Verification items for this drawing (mm, ordinates from the low corner). A direction names the side the tool comes from. Round coordinates to 2 decimals unless told otherwise and drop trailing zeros. Order: outer loops, then holes, each group sorted by start corner. A loop starts at its lowest first (then second) coordinate and runs counter-clockwise, first axis right, second up. Notation, with made-up numbers: (65, -15.5) - (89, -15.5) arc R23 ccw to (89, 15.5) - close; hole circle Ø3 at (-1, 60.25). An arc over 180 degrees is marked (long way). Return JSON: item names as keys, results as strings. Group by question number.
Q1. Material ranges on line 1 along Y through (x, z) = (3.75, 0.8); line 2 along X through (y, z) = (3.5, 1.4); line 3 along X through (y, z) = (12, 1.25), recorded low to high.
Q2. Sectioned sample at C-C, the plane y = 2.5. Record the cut outline in (x, z), then the cut area to 3 significant figures.
Q3. Sectioned sample at B-B, the plane x = 3. Record the cut outline in (y, z).
Q4. Sectioned sample at A-A, the plane z = 1.6. Record the cut outline in (x, y), then the cut area to 3 significant figures.
Q5. Tool access check on the marked faces 1, 2 and 3. Record the directions out of +Z, -Z, +X, -X, +Y, -Y that give a thin tool (end or side, any length) a straight path to the whole face; none if there is none.
Q6. Gauge pin test, flat ends, axial feed: pin 1 Ø0.6 at (y, z) = (2, 1) entering from +X; pin 2 Ø1.5 at (x, y) = (9.5, 4) entering from -Z. Record the tip position at first contact, or that the pin passes through.
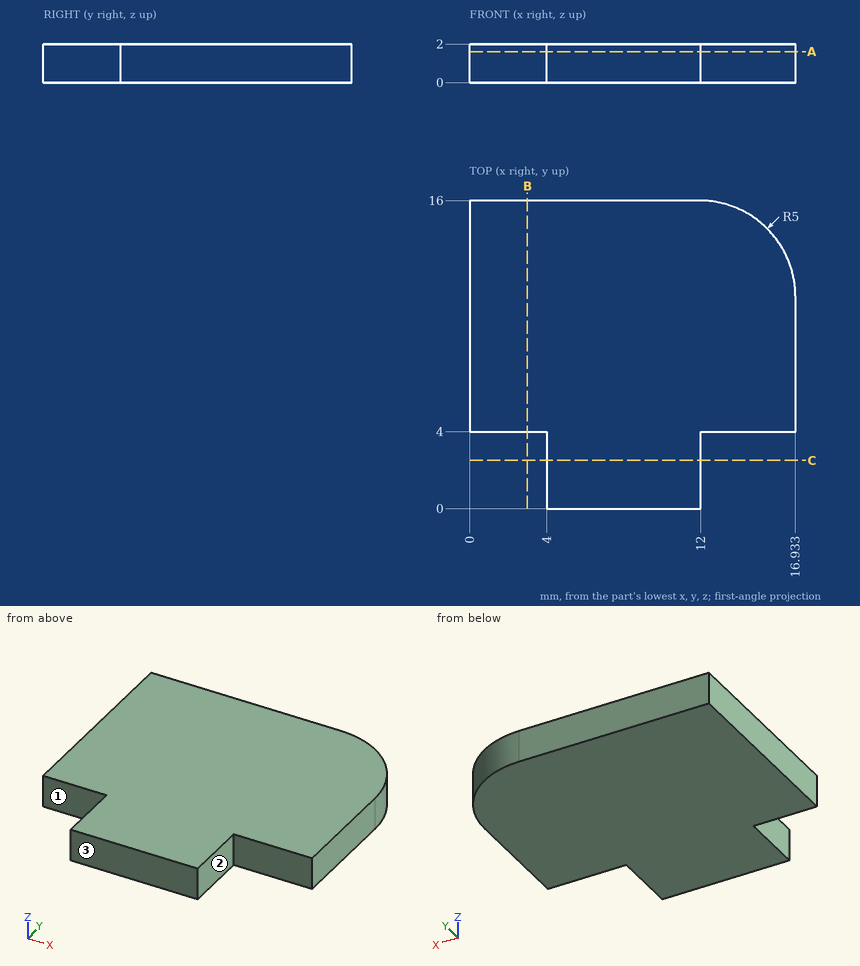
Reply:
{
 "1": {"line 1": "4 to 16", "line 2": "4 to 12", "line 3": "0 to 16.83"},
 "2": {"outline": "(4, 0) - (12, 0) - (12, 2) - (4, 2) - close", "area": "16.0 mm^2"},
 "3": {"outline": "(4, 0) - (16, 0) - (16, 2) - (4, 2) - close"},
 "4": {"outline": "(0, 4) - (4, 4) - (4, 0) - (12, 0) - (12, 4) - (16.93, 4) - (16.93, 11) arc R5 ccw to (11.93, 16) - (0, 16) - close", "area": "230 mm^2"},
 "5": {"face 1": "+Z, -Z, -X, -Y", "face 2": "+Z, -Z, +X, -Y", "face 3": "+Z, -Z, +X, -X, -Y"},
 "6": {"pin 1": "x = 12", "pin 2": "z = 0"}
}
